Verification items for the finished model (mm, model axes). Give positions to 0.01 mm unless a question says otherwise; leave off trailing zeros. Loops run counter-clockwise (first coordinate to the right, second up) from the corner with the lowest first, then second, coordinate; pieces in that order, holes last. Notation, with made-up numbers: M -27,54 L 32,54 A31 cw 32,83 Z; hole C 66.5,64 d2. An arc over 180 degrees is marked long. Put each result on its own line as item: value. Start each with the question number.
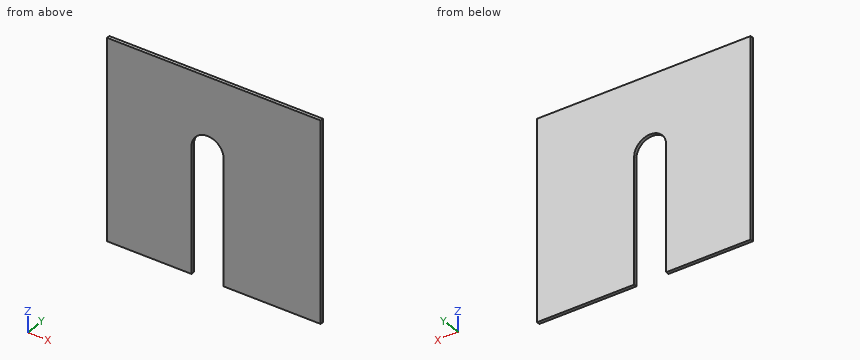
from build123d import *

# Parameters (mm, degrees)
F0_W     = 66.633955
F0_H     = 62.271908
F1_DEPTH = 1
F3_DEPTH = 1.001


with BuildPart() as f1:
    # F0 (on Front) → F1 (new body)
    with BuildSketch(Plane.XZ):
        with Locations((33.316978, 31.135954)):
            Rectangle(F0_W, F0_H)
    extrude(amount=F1_DEPTH)

    # F2 (on face) → F3 (cut, through all)
    with BuildSketch(Plane.XZ.offset(1)):
        with BuildLine():
            Line((31.349327, 0), (36.349327, 0))
            Line((36.349327, 0), (36.349327, 39.112926))
            ThreePointArc((36.349327, 39.112926), (31.349327, 44.112926), (26.349327, 39.112926))
            Line((26.349327, 39.112926), (26.349327, 0))
            Line((26.349327, 0), (31.349327, 0))
        make_face()
    extrude(amount=-F3_DEPTH, mode=Mode.SUBTRACT)


solid = f1.part
Q1. Cross-section at C-C, the plane z = 5. Record the boundary of the cut face in (x, y).
Q2. Cross-section at B-B, the plane y = -0.85. Record the boundary of the cut face in (x, z).
Q3. Cross-section at D-D, the plane x = 33. Record the boundary of the cut face in (y, z), then the cut area to 3 significant figures.
Q4. Cross-section at A-A, the plane z = 43. Record the boundary of the cut face in (x, y), then the cut area to 3 significant figures.
Q5. Scan lines: L1, parallel to X at y = -0.1, z = 9; L2, parallel to X at y = -0.35, z = 42; L3, parallel to Z at x = 34.5, y = -0.5. Record each from-to range of solid material in increasing order.
Ans:
1. outline: M 0,-1 L 26.35,-1 L 26.35,0 L 0,0 Z; M 36.35,-1 L 66.63,-1 L 66.63,0 L 36.35,0 Z
2. outline: M 0,0 L 26.35,0 L 26.35,39.11 A5 cw 36.35,39.11 L 36.35,0 L 66.63,0 L 66.63,62.27 L 0,62.27 Z
3. outline: M -1,43.83 L 0,43.83 L 0,62.27 L -1,62.27 Z
3. area: 18.4 mm^2
4. outline: M 0,-1 L 28.2,-1 L 28.2,0 L 0,0 Z; M 34.49,-1 L 66.63,-1 L 66.63,0 L 34.49,0 Z
4. area: 60.3 mm^2
5. L1: x = 0 to 26.35, 36.35 to 66.63
5. L2: x = 0 to 27.27, 35.43 to 66.63
5. L3: z = 43 to 62.27
